Design review of the part built by this model. Coordinates are the model's own, in mm. A direction names the side the tool comes from. Coordinates: 2 decimals unless noted, no trailing zeros. Loops run counter-clockwise (first coordinate to the right, second up) from the corner with the lowest first, then second, coordinate; pieces in that order, holes last. Notation, with made-up numbers: (22.25, 30) -> (71.25, 30) arc R23 cw to (71.25, 68) -> close; hole circle Ø2 at (-21, 17). An arc over 180 degrees is marked (long way). Answer in a Markdown table with one row per item.
```python
from build123d import *

# Parameters (mm, degrees)
PAD002_DEPTH = 1.4
FILLET_R     = 1
CHAMFER_SIZE = 1


with BuildPart() as part:
    # Sketch003 → Pad002 (new body)
    with BuildSketch(Plane.XY):
        with BuildLine():
            Line((-64.304214, 37.25), (64.304214, 37.25))
            ThreePointArc((73.3, 28.254214), (70.665195, 34.615195), (64.304214, 37.25))
            Line((73.3, 28.254214), (73.3, -28.254214))
            ThreePointArc((64.304214, -37.25), (70.665195, -34.615195), (73.3, -28.254214))
            Line((64.304214, -37.25), (-64.304214, -37.25))
            ThreePointArc((-73.3, -28.254214), (-70.665195, -34.615195), (-64.304214, -37.25))
            Line((-73.3, -28.254214), (-73.3, 28.254214))
            ThreePointArc((-64.304214, 37.25), (-70.665195, 34.615195), (-73.3, 28.254214))
        make_face()
        with BuildLine():
            Line((-61.82934, 33.75), (61.82934, 33.75))
            ThreePointArc((69.8, 25.77934), (67.465448, 31.415448), (61.82934, 33.75))
            Line((69.8, 25.77934), (69.8, -25.77934))
            ThreePointArc((61.82934, -33.75), (67.465448, -31.415448), (69.8, -25.77934))
            Line((61.82934, -33.75), (-61.82934, -33.75))
            ThreePointArc((-69.8, -25.77934), (-67.465448, -31.415448), (-61.82934, -33.75))
            Line((-69.8, -25.77934), (-69.8, 25.77934))
            ThreePointArc((-61.82934, 33.75), (-67.465448, 31.415448), (-69.8, 25.77934))
        make_face(mode=Mode.SUBTRACT)
    extrude(amount=PAD002_DEPTH)

    # Fillet
    fillet_edges = [part.edges().sort_by_distance(p)[0] for p in [
        (0, 33.75, 1.4),
        (-67.465448, 31.415448, 1.4),
        (-69.8, 0, 1.4),
        (-67.465448, -31.415448, 1.4),
        (0, -33.75, 1.4),
        (67.465448, -31.415448, 1.4),
        (69.8, 0, 1.4),
        (67.465448, 31.415448, 1.4),
    ]]
    fillet(fillet_edges, radius=FILLET_R)

    # Chamfer
    chamfer_edges = [part.edges().sort_by_distance(p)[0] for p in [
        (0, 37.25, 1.4),
        (70.665195, 34.615195, 1.4),
        (73.3, 0, 1.4),
        (70.665195, -34.615195, 1.4),
        (0, -37.25, 1.4),
        (-70.665195, -34.615195, 1.4),
        (-73.3, 0, 1.4),
        (-70.665195, 34.615195, 1.4),
    ]]
    chamfer(chamfer_edges, length=CHAMFER_SIZE)


solid = part.part
```
(1) Take a section at C-C on z = 0.7. Give the boundary of the cut face in (x, y).
Evaluation:
| item | result |
|---|---|
| outline | (-73, -28.25) arc R8.7 ccw to (-64.3, -36.95) -> (64.3, -36.95) arc R8.7 ccw to (73, -28.25) -> (73, 28.25) arc R8.7 ccw to (64.3, 36.95) -> (-64.3, 36.95) arc R8.7 ccw to (-73, 28.25) -> close; hole (-69.85, -25.78) arc R8.02 ccw to (-61.83, -33.8) -> (61.83, -33.8) arc R8.02 ccw to (69.85, -25.78) -> (69.85, 25.78) arc R8.02 ccw to (61.83, 33.8) -> (-61.83, 33.8) arc R8.02 ccw to (-69.85, 25.78) -> close |
(2) Draft analysis for pull direction X (two halves, no side actions). For faces 3 (the cylindrical face through (67.53, 31.35, 0.2)), 4 (the cylindrical face through (70.735, 34.545, 0.197)), 5 (the flat face through (0, 35, 1.4)), state which applies: pulls with the +X half, pulls with the -X half, needs draft (parallel to the pull), parting line crosses it, or undercut.
Evaluation:
| item | result |
|---|---|
| face 3 | undercut |
| face 4 | pulls with the +X half |
| face 5 | needs draft |
(3) Tool access review of faces 1 (the cylindrical face through (-67.53, -31.35, 0.2)), 2 (the conical face through (-70.144, 33.967, 1.226)): name each direction out of +Z, -Z, +X, -X, +Y, -Y from which nothing blocks a thin tool from reaching the whole face with its end or side.
Evaluation:
| item | result |
|---|---|
| face 1 | +Z, -Z |
| face 2 | +Z, -X, +Y |
(4) To check wall thickness, follow probe 1 along Y at (x, z) = (16, 0.25); probe 2 along X at (y, z) = (22.5, 0.95). State the ranges of each line that lie inside material, in increasing order.
Evaluation:
| item | result |
|---|---|
| probe 1 | y = -37.25 to -33.75, 33.75 to 37.25 |
| probe 2 | x = -72.75 to -69.96, 69.96 to 72.75 |
(5) Take a section at B-B on y = -10. Give the boundary of the cut face in (x, z), and give its area (3 significant figures).
Evaluation:
| item | result |
|---|---|
| outline | (-73.3, 0) -> (-69.8, 0) -> (-69.8, 0.4) arc R1 ccw to (-70.8, 1.4) -> (-72.3, 1.4) -> (-73.3, 0.4) -> close; (69.8, 0) -> (73.3, 0) -> (73.3, 0.4) -> (72.3, 1.4) -> (70.8, 1.4) arc R1 ccw to (69.8, 0.4) -> close |
| area | 8.37 mm² |
(6) Take a section at A-A on x = -13.5. Give the boundary of the cut face in (y, z).
Evaluation:
| item | result |
|---|---|
| outline | (-37.25, 0) -> (-33.75, 0) -> (-33.75, 0.4) arc R1 ccw to (-34.75, 1.4) -> (-36.25, 1.4) -> (-37.25, 0.4) -> close; (33.75, 0) -> (37.25, 0) -> (37.25, 0.4) -> (36.25, 1.4) -> (34.75, 1.4) arc R1 ccw to (33.75, 0.4) -> close |
